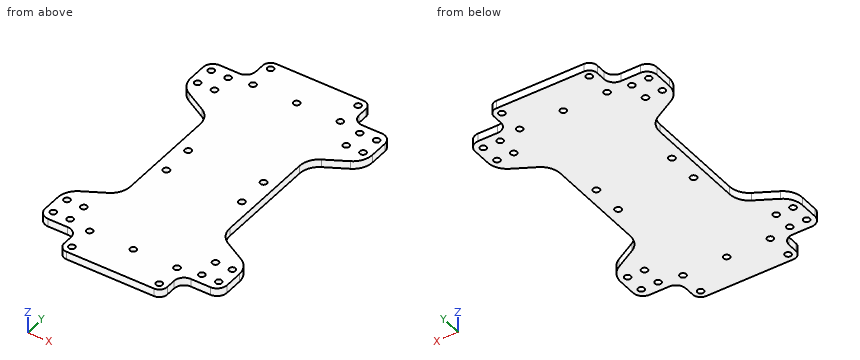
from build123d import *

# Parameters (mm, degrees)
SKETCH1_R           = 1.6
SKETCH1_R_2         = 1.65
BOSS_EXTRUDE1_DEPTH = 4
FILLET2_R           = 10
FILLET3_R           = 5


with BuildPart() as part:
    # Sketch1 → Boss-Extrude1 (new body)
    with BuildSketch(Plane.XY):
        with BuildLine():
            Line((1.40773023, -0.063608297), (16.206941284, -0.063608297))
            ThreePointArc((16.206941284, -0.063608297), (19.74247519, -1.528074391), (21.206941284, -5.063608297))
            Line((21.206941284, -5.063608297), (21.206941284, -10.063608297))
            ThreePointArc((21.206941284, -10.063608297), (22.37851416, -12.892035422), (25.206941284, -14.063608297))
            Line((25.206941284, -14.063608297), (69.208519176, -14.063608297))
            ThreePointArc((69.208519176, -14.063608297), (72.036946301, -12.892035422), (73.208519176, -10.063608297))
            Line((73.208519176, -10.063608297), (73.208519176, -5.063608297))
            ThreePointArc((73.208519176, -5.063608297), (74.67298527, -1.528074391), (78.208519176, -0.063608297))
            Line((78.208519176, -0.063608297), (93.00773023, -0.063608297))
            Line((93.00773023, -0.063608297), (93.00773023, 19.936391703))
            Line((93.00773023, 19.936391703), (72.20773023, 31.430017028))
            Line((72.20773023, 31.430017028), (72.20773023, 94.442766377))
            Line((72.20773023, 94.442766377), (93.00773023, 105.936391703))
            Line((93.00773023, 105.936391703), (93.00773023, 125.936391703))
            Line((93.00773023, 125.936391703), (78.208519176, 125.936391703))
            ThreePointArc((78.208519176, 125.936391703), (74.67298527, 127.400857797), (73.208519176, 130.936391703))
            Line((73.208519176, 130.936391703), (73.208519176, 135.936391703))
            ThreePointArc((73.208519176, 135.936391703), (72.036946301, 138.764818827), (69.208519176, 139.936391703))
            Line((69.208519176, 139.936391703), (25.206941284, 139.936391703))
            ThreePointArc((25.206941284, 139.936391703), (22.37851416, 138.764818827), (21.206941284, 135.936391703))
            Line((21.206941284, 135.936391703), (21.206941284, 130.936391703))
            ThreePointArc((21.206941284, 130.936391703), (19.74247519, 127.400857797), (16.206941284, 125.936391703))
            Line((16.206941284, 125.936391703), (1.40773023, 125.936391703))
            Line((1.40773023, 125.936391703), (1.40773023, 105.936391703))
            Line((1.40773023, 105.936391703), (22.20773023, 94.442766377))
            Line((22.20773023, 94.442766377), (22.20773023, 31.430017028))
            Line((22.20773023, 31.430017028), (1.40773023, 19.936391703))
            Line((1.40773023, 19.936391703), (1.40773023, -0.063608297))
        make_face()
        with Locations((5.55773023, 4.936391703)):
            Circle(SKETCH1_R, mode=Mode.SUBTRACT)
        with Locations((14.05773023, 4.936391703)):
            Circle(SKETCH1_R, mode=Mode.SUBTRACT)
        with Locations((14.05773023, 14.936391703)):
            Circle(SKETCH1_R, mode=Mode.SUBTRACT)
        with Locations((5.55773023, 14.936391703)):
            Circle(SKETCH1_R, mode=Mode.SUBTRACT)
        with Locations(Location((69.208519176, -10.063608297, 0), (0, 0, 180))):
            Circle(SKETCH1_R, mode=Mode.SUBTRACT)
        with Locations(Location((69.208519176, 2.936391703, 0), (0, 0, 180))):
            Circle(SKETCH1_R, mode=Mode.SUBTRACT)
        with Locations((47.206941284, 2.936391703)):
            Circle(SKETCH1_R, mode=Mode.SUBTRACT)
        with Locations(Location((66.20773023, 54.936391703, 0), (0, 0, 180))):
            Circle(SKETCH1_R_2, mode=Mode.SUBTRACT)
        with Locations(Location((88.85773023, 14.936391703, 0), (0, 0, 180))):
            Circle(SKETCH1_R, mode=Mode.SUBTRACT)
        with Locations(Location((80.35773023, 14.936391703, 0), (0, 0, 180))):
            Circle(SKETCH1_R, mode=Mode.SUBTRACT)
        with Locations(Location((80.35773023, 4.936391703, 0), (0, 0, 180))):
            Circle(SKETCH1_R, mode=Mode.SUBTRACT)
        with Locations(Location((88.85773023, 4.936391703, 0), (0, 0, 180))):
            Circle(SKETCH1_R, mode=Mode.SUBTRACT)
        with Locations((28.20773023, 54.936391703)):
            Circle(SKETCH1_R_2, mode=Mode.SUBTRACT)
        with Locations(Location((25.206941284, 135.936391703, 0), (0, 0, 180))):
            Circle(SKETCH1_R, mode=Mode.SUBTRACT)
        with Locations((25.206941284, 2.936391703)):
            Circle(SKETCH1_R, mode=Mode.SUBTRACT)
        with Locations(Location((25.206941284, 122.936391703, 0), (0, 0, 180))):
            Circle(SKETCH1_R, mode=Mode.SUBTRACT)
        with Locations(Location((28.20773023, 70.936391703, 0), (0, 0, 180))):
            Circle(SKETCH1_R_2, mode=Mode.SUBTRACT)
        with Locations((25.206941284, -10.063608297)):
            Circle(SKETCH1_R, mode=Mode.SUBTRACT)
        with Locations((88.85773023, 120.936391703)):
            Circle(SKETCH1_R, mode=Mode.SUBTRACT)
        with Locations((80.35773023, 120.936391703)):
            Circle(SKETCH1_R, mode=Mode.SUBTRACT)
        with Locations((80.35773023, 110.936391703)):
            Circle(SKETCH1_R, mode=Mode.SUBTRACT)
        with Locations((88.85773023, 110.936391703)):
            Circle(SKETCH1_R, mode=Mode.SUBTRACT)
        with Locations((66.20773023, 70.936391703)):
            Circle(SKETCH1_R_2, mode=Mode.SUBTRACT)
        with Locations(Location((47.206941284, 122.936391703, 0), (0, 0, 180))):
            Circle(SKETCH1_R, mode=Mode.SUBTRACT)
        with Locations((69.208519176, 122.936391703)):
            Circle(SKETCH1_R, mode=Mode.SUBTRACT)
        with Locations((69.208519176, 135.936391703)):
            Circle(SKETCH1_R, mode=Mode.SUBTRACT)
        with Locations(Location((5.55773023, 110.936391703, 0), (0, 0, 180))):
            Circle(SKETCH1_R, mode=Mode.SUBTRACT)
        with Locations(Location((14.05773023, 110.936391703, 0), (0, 0, 180))):
            Circle(SKETCH1_R, mode=Mode.SUBTRACT)
        with Locations(Location((14.05773023, 120.936391703, 0), (0, 0, 180))):
            Circle(SKETCH1_R, mode=Mode.SUBTRACT)
        with Locations(Location((5.55773023, 120.936391703, 0), (0, 0, 180))):
            Circle(SKETCH1_R, mode=Mode.SUBTRACT)
    extrude(amount=BOSS_EXTRUDE1_DEPTH)

    # Fillet2
    fillet2_edges = [part.edges().sort_by_distance(p)[0] for p in [
        (1.40773023, 19.936391703, 2),
        (22.20773023, 31.430017028, 2),
        (22.20773023, 94.442766377, 2),
        (1.40773023, 105.936391703, 2),
        (93.00773023, 105.936391703, 2),
        (72.20773023, 94.442766377, 2),
        (72.20773023, 31.430017028, 2),
        (93.00773023, 19.936391703, 2),
    ]]
    fillet(fillet2_edges, radius=FILLET2_R)

    # Fillet3
    fillet3_edges = [part.edges().sort_by_distance(p)[0] for p in [
        (1.40773023, 125.936391703, 2),
        (93.00773023, 125.936391703, 2),
        (93.00773023, -0.063608297, 2),
        (1.40773023, -0.063608297, 2),
    ]]
    fillet(fillet3_edges, radius=FILLET3_R)


solid = part.part
Model file for the job. Use its own axes, mm. Coordinates: 2 decimals unless noted, no trailing zeros. Order: outer loops, then holes, each group sorted by start corner. A loop starts at its lowest first (then second) coordinate and runs counter-clockwise, first axis right, second up. Notation, with made-up numbers: M 8,-27 L 42,-27 A13 ccw 42,-9 Z; hole C 69,32.5 d8. An arc over 180 degrees is marked long. Return JSON: item names as keys, results as strings.
1. Flat gauge pins, fed straight in: pin 1 (2 mm diameter, centred on y = 25.5, z = 0.5, fed in from -X); pin 2 (2 mm diameter, centred on x = 81.5, z = 1.5, fed in from -Y); pin 3 (1.2 mm diameter, centred on y = 71, z = 1.5, fed in from -X). Where does each tip first touch, or does it go through?
Ans:
{"pin 1": "x = 9.67", "pin 2": "y = -0.06", "pin 3": "x = 22.21"}
2. Saw through at B-B (z = 3.3). Give the number of separate pieces and of enclosed holes in the cut face, and give its area (3 significant figures).
Ans:
{"separate pieces": "1", "enclosed holes": "30", "area": "9,640 mm^2"}
3. Saw through at C-C (y = 19.5). Give the cut face in (x, z).
Ans:
{"outline": "M 3.03,0 L 91.38,0 L 91.38,4 L 3.03,4 Z"}
4. Saw through at A-A (y = 49.5). Give the cut face in (x, z), and give its area (3 significant figures).
Ans:
{"outline": "M 22.21,0 L 72.21,0 L 72.21,4 L 22.21,4 Z", "area": "200 mm^2"}
5. Drill centre lines: probe 1 along Y at (x, z) = (66, 1.25); probe 2 along Y at (x, z) = (88, 1.35); probe 3 along Y at (x, z) = (87.5, 0.5). Where is each one in solid material? Low to high.
Ans:
{"probe 1": "-14.06 to 53.3, 56.57 to 69.3, 72.57 to 139.94", "probe 2": "-0.06 to 3.59, 6.29 to 13.59, 16.29 to 22.7, 103.17 to 109.59, 112.29 to 119.59, 122.29 to 125.94", "probe 3": "-0.06 to 4.09, 5.78 to 14.09, 15.78 to 22.98, 102.89 to 110.09, 111.78 to 120.09, 121.78 to 125.94"}
